```python
from build123d import *

# Parameters (mm, degrees)
PAD_DEPTH    = 10
SKETCH001_R  = 1.5
PAD001_DEPTH = 6
SKETCH002_R  = 1.5
POCKET_DEPTH = 8


with BuildPart() as part:
    # Sketch → Pad (new body)
    with BuildSketch(Plane.XY):
        Polygon((1.587713, -2.75), (3.175426, 0), (1.587713, 2.75), (-1.587713, 2.75), (-3.175426, 0), (-1.587713, -2.75), align=None)
    extrude(amount=PAD_DEPTH)

    # Sketch001 (on Face8 of Pad) → Pad001 (join)
    with BuildSketch(Plane.XY.offset(10)):
        Circle(SKETCH001_R)
    extrude(amount=PAD001_DEPTH)

    # Sketch002 (on Face4 of Pad001) → Pocket (cut)
    with BuildSketch(Plane(origin=(0, 0, 0), x_dir=(1, 0, 0), z_dir=(0, 0, -1))):
        Circle(SKETCH002_R)
    extrude(amount=-POCKET_DEPTH, mode=Mode.SUBTRACT)


solid = part.part
```
For this review, take the finished solid that the model builds, in its own axes (mm). A direction names the side the tool comes from. Coordinates: 2 decimals unless noted, no trailing zeros. Write each loop counter-clockwise with the first axis right and the second up, starting at its lowest first coordinate (ties: lowest second). Pieces come first, ordered by that corner, then holes. Notation, with made-up numbers: (-18.75, 72) - (-9.75, 72) arc R20 cw to (-9.75, 97) - close; hole circle Ø2 at (55, -22). An arc over 180 degrees is marked (long way). Put each result on its own line as item: value.
1. Add section A-A, the plane z = 3. Give the boundary of the cut face in (x, y).
Values found:
outline: (-3.18, 0) - (-1.59, -2.75) - (1.59, -2.75) - (3.18, 0) - (1.59, 2.75) - (-1.59, 2.75) - close; hole circle Ø3 at (0, 0)
2. For pin 1 (2.5 mm diameter, centred on x = 0, y = 0, fed in from -Z); pin 2 (2 mm diameter, centred on x = 0, z = 13.5, fed in from -Y); pin 3 (1 mm diameter, centred on x = 2.5, y = -2, fed in from +Z), all flat-tipped, find the tip position at first contact; note any pin that passes through.
Values found:
pin 1: z = 8
pin 2: y = -1.5
pin 3: z = 10
3. Wall thickness on probe 1 along Y at (x, z) = (0, 4.25); probe 2 along Z at (x, y) = (-1.75, 0.8); probe 3 along Z at (x, y) = (0.75, -1.1): over which ranges is each line inside the solid? List them lowest first.
Values found:
probe 1: -2.75 to -1.5, 1.5 to 2.75
probe 2: 0 to 10
probe 3: 8 to 16
4. Mouldability with a two-part tool opening along X and no side actions: class faces 1 (the cylindrical face through (-1.5, -0.07, 3.94)), 2 (the flat face through (2.37, -1.394, 4.93)), 3 (the flat face through (1.4, 1.3, 10)), 4 (the flat face through (-2.37, 1.394, 4.93)) as released by +X, released by -X, zero draft, split by the parting line, or undercut.
Values found:
face 1: undercut
face 2: released by +X
face 3: zero draft
face 4: released by -X
5. Add section B-B, the plane z = 9.5. Give the boundary of the cut face in (x, y).
Values found:
outline: (-3.18, 0) - (-1.59, -2.75) - (1.59, -2.75) - (3.18, 0) - (1.59, 2.75) - (-1.59, 2.75) - close
6. Add section D-D, the plane y = -1.1. Give the boundary of the cut face in (x, z), then the cut area to 3 significant figures.
Values found:
outline: (-2.54, 0) - (-1.02, 0) - (-1.02, 8) - (1.02, 8) - (1.02, 0) - (2.54, 0) - (2.54, 10) - (1.02, 10) - (1.02, 16) - (-1.02, 16) - (-1.02, 10) - (-2.54, 10) - close
area: 46.7 mm²
7. Add section C-C, the plane x = 0. Give the boundary of the cut face in (y, z).
Values found:
outline: (-2.75, 0) - (-1.5, 0) - (-1.5, 8) - (1.5, 8) - (1.5, 0) - (2.75, 0) - (2.75, 10) - (1.5, 10) - (1.5, 16) - (-1.5, 16) - (-1.5, 10) - (-2.75, 10) - close
8. Machinability: for faces 5 (the cylindrical face through (-1.5, 0.07, 12.96)), 6 (the flat face through (2.39, 1.36, 4.93)), 7 (the flat face through (0, 0, 8)), which of the approach directions +Z, -Z, +X, -X, +Y, -Y give a long, thin tool a straight path to every point of the face, cutting with its end or side? Answer none if there is none.
Values found:
face 5: +Z
face 6: +Z, -Z, +X, +Y
face 7: -Z
